Build history of the part. All positions in model axes, mm. A direction names the side the tool comes from. Round coordinates to 2 decimals unless told otherwise and drop trailing zeros. Loops run counter-clockwise (first coordinate to the right, second up) from the corner with the lowest first, then second, coordinate; pieces in that order, holes last. Notation, with made-up numbers: (34.25, 24.25) - (52.25, 24.25) arc R33 cw to (52.25, 61.25) - close; hole circle Ø11 at (-32, 15). An arc over 180 degrees is marked (long way). Use one line per item in the form item = value. Start each with the question number.
Q1. Mould opens along Y. For faces 1 (the face through (-24, -19, 10)), 2 (the face through (-11, -26, 2)), 3 (the face through (-15, -9.75, 5)) say: released by +Y, released by -Y, zero draft, split by the parting line, or undercut.
Q2. Saw through at D-D (x = -29). Give the cut face in (y, z), then the cut area to 3 significant figures.
Q3. Pin check, flat tips, straight feed: pin 1 (2.5 mm diameter, centred on x = -29.82, y = -29.75, fed in from +Z); pin 2 (15 mm diameter, centred on x = -14.82, y = -22.25, fed in from +Z). Stop position of each tip, or through.
Q4. Saw through at C-C (y = -26.5). Give the cut face in (x, z).
Q5. Drill centre lines: line 1 (Y direction, x = -15, z = 2.5); line 2 (Y direction, x = -31, z = 7.5); line 3 (Y direction, x = -0.5, z = 8). Where is each one in solid material? Low to high.
Q6. 3-axis set-ups, long thin cutter, end or side, ignore diameter. For faces 4 (the face through (-21.8, -15.8, 5.9)), 5 (the face through (-30.084, -12.767, 4.93)): which of +Z, -Z, +X, -X, +Y, -Y reach the whole face in a straight line?
Q7. Saw through at A-A (y = -16). Give the cut face in (x, z), then the cut area to 3 significant figures.
Q8. Saw through at B-B (z = 8.5). Give the cut face in (x, y), then the cut area to 3 significant figures.
```python
from build123d import *

# Parameters (mm, degrees)
ESQUISSE1_W        = 40
ESQUISSE1_H        = 25
ESQUISSE1_R        = 9.5
ESQUISSE1_R_2      = 2
BOSS_EXTRU_1_DEPTH = 10
ESQUISSE1_4_R      = 9.5
ESQUISSE1_4_R_2    = 5
BOSS_EXTRU_2_DEPTH = 2


with BuildPart() as part:
    # Esquisse1 → Boss.-Extru.1 (new body)
    with BuildSketch(Plane.XY):
        with Locations((-14.823595047, -22.249813872)):
            Rectangle(ESQUISSE1_W, ESQUISSE1_H)
        with Locations((-14.823595047, -22.249813872)):
            Circle(ESQUISSE1_R, mode=Mode.SUBTRACT)
        with Locations((0.176404953, -29.749813872)):
            Circle(ESQUISSE1_R_2, mode=Mode.SUBTRACT)
        with Locations((0.176404953, -14.749813872)):
            Circle(ESQUISSE1_R_2, mode=Mode.SUBTRACT)
        with Locations((-29.823595047, -29.749813872)):
            Circle(ESQUISSE1_R_2, mode=Mode.SUBTRACT)
        with Locations((-29.823595047, -14.749813872)):
            Circle(ESQUISSE1_R_2, mode=Mode.SUBTRACT)
    extrude(amount=BOSS_EXTRU_1_DEPTH)

    # Esquisse1_4 → Boss.-Extru.2 (add)
    with BuildSketch(Plane.XY):
        with Locations((-14.823595047, -22.249813872)):
            Circle(ESQUISSE1_4_R)
        with Locations((-14.823595047, -22.249813872)):
            Circle(ESQUISSE1_4_R_2, mode=Mode.SUBTRACT)
    extrude(amount=BOSS_EXTRU_2_DEPTH)


solid = part.part
```
Report:
q1.face_1 = zero draft
q1.face_2 = undercut
q1.face_3 = released by +Y
q2.outline = (-34.75, 0) - (-31.57, 0) - (-31.57, 10) - (-34.75, 10) - close; (-27.93, 0) - (-16.57, 0) - (-16.57, 10) - (-27.93, 10) - close; (-12.93, 0) - (-9.75, 0) - (-9.75, 10) - (-12.93, 10) - close
q2.area = 177 mm²
q3.pin_1 = through
q3.pin_2 = 2
q4.outline = (-34.82, 0) - (-17.46, 0) - (-17.46, 2) - (-23.32, 2) - (-23.32, 10) - (-34.82, 10) - close; (-12.19, 0) - (5.18, 0) - (5.18, 10) - (-6.33, 10) - (-6.33, 2) - (-12.19, 2) - close
q5.line_1 = -34.75 to -31.75, -12.75 to -9.75
q5.line_2 = -34.75 to -31.37, -28.13 to -16.37, -13.13 to -9.75
q5.line_3 = -34.75 to -31.63, -27.87 to -16.63, -12.87 to -9.75
q6.face_4 = +Z
q6.face_5 = +Z, -Z
q7.outline = (-34.82, 0) - (-31.38, 0) - (-31.38, 10) - (-34.82, 10) - close; (-28.26, 0) - (-1.38, 0) - (-1.38, 10) - (-7.67, 10) - (-7.67, 2) - (-21.98, 2) - (-21.98, 10) - (-28.26, 10) - close; (1.74, 0) - (5.18, 0) - (5.18, 10) - (1.74, 10) - close
q7.area = 223 mm²
q8.outline = (-34.82, -34.75) - (5.18, -34.75) - (5.18, -9.75) - (-34.82, -9.75) - close; hole circle Ø4 at (-29.82, -29.75); hole circle Ø4 at (-29.82, -14.75); hole circle Ø19 at (-14.82, -22.25); hole circle Ø4 at (0.18, -29.75); hole circle Ø4 at (0.18, -14.75)
q8.area = 666 mm²
